Autodesk Inventor part; units mm, degrees
ref_plane "YZ Plane" through (0, 0, 0) normal (1, 0, 0) x (0, 1, 0)
ref_plane "XZ Plane" through (0, 0, 0) normal (0, 1, 0) x (-1, 0, 0)
ref_plane "XY Plane" through (0, 0, 0) normal (0, 0, 1) x (1, 0, 0)
sketch "Sketch1" plane through (0, 0, 0) normal (0, 0, 1) x (1, 0, 0)
  line L0 (0, 0) -> (38.5, 0)
  line L1 (0, 0) -> (0, 48)
  line L2 (0, 48) -> (38.5, 48)
  line L3 (38.5, 48) -> (38.5, 0)
  circle A0 centre (9.25, 18) radius 2.25
  line L4 (9.25, 18) -> (29.25, 18)
  circle A1 centre (29.25, 18) radius 2.25
  circle A2 centre (9.25, 36) radius 2.25
  line L5 (9.25, 36) -> (29.25, 36)
  circle A3 centre (29.25, 36) radius 2.25
  dimension "d0" = 48
  dimension "d3" = 18
  dimension "d4" = 4.5
  dimension "d5" = 4.5
  dimension "d6" = 20
  dimension "d7" = 38.5
  dimension "d8" = 9.25
  dimension "d9" = 4.5
  dimension "d10" = 4.5
  dimension "d11" = 20
  dimension "d12" = 12
  dimension "d13" = 9.25
extrude "Extrusion1" add sketch "Sketch1" along normal blind 6
equation "\"d5\" = d4"
equation "\"d8\" = -0.5 * d6 + 0.5 * d7"
equation "\"d10\" = d9"
equation "\"d13\" = -0.5 * d11 + 0.5 * d7"
properties part number "BaseC_9" material "PMMA Plastic"
Model file for the job. Use its own axes, mm. Round coordinates to 2 decimals unless told otherwise and drop trailing zeros. Write each loop counter-clockwise with the first axis right and the second up, starting at its lowest first coordinate (ties: lowest second). Pieces come first, ordered by that corner, then holes. Notation, with made-up numbers: (-33, 49) -> (-14, 49) arc R7 cw to (-14, 62) -> close; hole circle Ø5 at (6.5, 0.5). An arc over 180 degrees is marked (long way). Answer as CSV lines item,"result".
1. Slice it at A-A, the plane x = 29.25. List the corners of the cut face in (y, z).
Resolved:
outline,"(0, 0) -> (15.75, 0) -> (15.75, 6) -> (0, 6) -> close; (20.25, 0) -> (33.75, 0) -> (33.75, 6) -> (20.25, 6) -> close; (38.25, 0) -> (48, 0) -> (48, 6) -> (38.25, 6) -> close"
2. Pin check, flat tip, straight feed: pin 1 Ø3.5 at (x, y) = (9.25, 36) entering from +Z. Stop position of the tip, or through.
Resolved:
pin 1,"through"
3. Drill centre lines: line 1 (Y direction, x = 9.25, z = 2.65); line 2 (X direction, y = 18.5, z = 0.3); line 3 (Y direction, x = 8.5, z = 0.65). Where is each one in solid material? Low to high.
Resolved:
line 1,"0 to 15.75, 20.25 to 33.75, 38.25 to 48"
line 2,"0 to 7.06, 11.44 to 27.06, 31.44 to 38.5"
line 3,"0 to 15.88, 20.12 to 33.88, 38.12 to 48"
4. Slice it at C-C, the plane y = 36. List the corners of the cut face in (x, z).
Resolved:
outline,"(0, 0) -> (7, 0) -> (7, 6) -> (0, 6) -> close; (11.5, 0) -> (27, 0) -> (27, 6) -> (11.5, 6) -> close; (31.5, 0) -> (38.5, 0) -> (38.5, 6) -> (31.5, 6) -> close"
5. Mould opens along Y. For faces 1 (the face through (38.5, 24, 3)), 2 (the face through (8.762, 20.196, 2.958)), 3 (the face through (19, 0, 3)) say: +Y half, -Y half, draft (parallel to the pull), parting line (faces both ways), or undercut.
Resolved:
face 1,"draft"
face 2,"undercut"
face 3,"-Y half"
6. Slice it at B-B, the plane z = 0.85. List the corners of the cut face in (x, y), plus the area to 3 significant figures.
Resolved:
outline,"(0, 0) -> (38.5, 0) -> (38.5, 48) -> (0, 48) -> close; hole circle Ø4.5 at (9.25, 18); hole circle Ø4.5 at (9.25, 36); hole circle Ø4.5 at (29.25, 18); hole circle Ø4.5 at (29.25, 36)"
area,"1,780 mm²"
